Design review of the part built by this model. Coordinates are the model's own, in mm. A direction names the side the tool comes from. Give positions to 0.01 mm unless a question says otherwise; leave off trailing zeros. Loops run counter-clockwise (first coordinate to the right, second up) from the corner with the lowest first, then second, coordinate; pieces in that order, holes last. Notation, with made-up numbers: (12.5, 80) -> (47.5, 80) arc R14 cw to (47.5, 90) -> close; hole circle Ø5 at (45.5, 25.25). An arc over 180 degrees is marked (long way). Answer in a Markdown table with one row per item. Add a question column.
(1) Draft analysis for pull direction Y (two halves, no side actions). For faces 1 (the flat face through (3.763, 2.213, 2.442)), 2 (the cylindrical face through (-0.34, -1.55, 5.38)), 3 (the cylindrical face through (0.632, -1.525, 2.479)), 4 (the flat face through (0, -4.366, 2)), state which applies: +Y half, -Y half, draft (parallel to the pull), parting line (faces both ways), or undercut.
(2) For faces 5 (the flat face through (2, 0, 0)), 6 (the flat face through (0, -2, 5.715)), list the 3-axis set-ups (+Z, -Z, +X, -X, +Y, -Y) from which the entire face can be reached by the end or side of a thin tool; tool diameter is ignored.
(3) For line 1 (Y direction, x = 0, z = 2.1); line 2 (Y direction, x = 1.25, z = 5.45); line 3 (X direction, y = 1.5, z = 4.4), list the stretches that pass through material, from the lowest coordinate up.
(4) Consider section B-B on z = 0.55. Write out the cut boundary in (x, y), then the cut area to 3 significant figures.
(5) Consider section C-C on z = 5.55. Write out the cut boundary in (x, y) (1 decimal).
(6) For pin 1 (1.5 mm diameter, centred on x = 3.5, z = 2.5, fed in from +Y); pin 2 (1.7 mm diameter, centred on x = 0.5, y = 0, fed in from -Z); pin 3 (1 mm diameter, centred on y = -1.5, z = 1, fed in from -X); pin 4 (2.5 mm diameter, centred on x = 0, y = 0.5, fed in from +Z) (3 decimals), all flat-tipped, find the tip position at first contact; note any pin that passes through.
Autodesk Inventor part; units mm, degrees
ref_plane "YZ Plane" through (0, 0, 0) normal (1, 0, 0) x (0, 1, 0)
ref_plane "XZ Plane" through (0, 0, 0) normal (0, 1, 0) x (-1, 0, 0)
ref_plane "XY Plane" through (0, 0, 0) normal (0, 0, 1) x (1, 0, 0)
sketch "Sketch1" plane through (0, 0, 0) normal (0, 0, 1) x (1, 0, 0)
  line L0 (-2.5205, 4.3656) -> (2.5205, 4.3656)
  line L1 (2.5205, 4.3656) -> (5.041, 0)
  line L2 (5.041, 0) -> (2.5205, -4.3656)
  line L3 (2.5205, -4.3656) -> (-2.5205, -4.3656)
  line L4 (-2.5205, -4.3656) -> (-5.041, 0)
  line L5 (-5.041, 0) -> (-2.5205, 4.3656)
  point P0 (0, 0)
  point P1 (0, 0)
  dimension "d0" = 8.7312
extrude "Extrusion1" add sketch "Sketch1" along normal blind 4.953
sketch "Sketch2" plane through (0, 0, 0) normal (1, 0, 0) x (0, 1, 0)
  line L0 (4.3656, 4.953) -> (4.3656, 0) construction
  line L1 (4.3656, 0) -> (-4.3656, 0) construction
  line L2 (-4.3656, 0) -> (-4.3656, 4.953) construction
  line L3 (-4.3656, 4.953) -> (4.3656, 4.953) construction
  line L4 (0, 4.953) -> (0, 5.9436)
  line L5 (-4.3656, 4.953) -> (0, 4.953)
  arc A0 (-3.3782, 5.9436) -> (-4.3688, 4.953) centre (-3.3782, 4.953) ccw
  line L6 (-3.3782, 5.9436) -> (0, 5.9436)
  line L7 (0, 5.9436) -> (0, 4.953)
  line L8 (0, 4.953) -> (-4.3688, 4.953)
  point P0 (0, 0)
  dimension "d6" = 0.9906
  dimension "d7" = 3.3782
revolve "Revolution1" add sketch "Sketch2" angle 360 about axis through (0, 0, 4.953) along (0, 0, 1)
sketch "Sketch3" plane through (0, 0, 0) normal (0, 1, 0) x (-1, 0, 0)
  arc A0 (-3.3782, 5.9436) -> (-4.3688, 4.953) centre (-3.3782, 4.953) ccw construction
  line L0 (-3.3782, 5.9436) -> (3.3782, 5.9436) construction
  arc A1 (4.3688, 4.953) -> (3.3782, 5.9436) centre (3.3782, 4.953) ccw construction
  line L1 (4.3688, 4.953) -> (5.041, 4.953) construction
  line L2 (5.041, 4.953) -> (5.041, 0) construction
  line L3 (5.041, 0) -> (-5.041, 0) construction
  line L4 (-5.041, 0) -> (-5.041, 4.953) construction
  line L5 (-5.041, 4.953) -> (-4.3688, 4.953) construction
  line L6 (-4.3552, 4.953) -> (-5.041, 4.6482)
  line L7 (-5.041, 4.6482) -> (-5.041, 4.953)
  line L8 (-5.041, 4.953) -> (-4.3552, 4.953)
  line L9 (0, 0) -> (0, 7.4764) construction
  line L10 (-5.041, 0.3048) -> (-4.3552, 0)
  line L11 (-5.041, 0.3048) -> (-5.041, 0)
  line L12 (-5.041, 0) -> (-4.3552, 0)
  dimension "d9" = 0.6858
  dimension "d10" = 0.3048
  dimension "d11" = 0.3048
  dimension "d12" = 0.6858
revolve "Revolution2" cut sketch "Sketch3" angle 360 about axis through (0, 0, 0) along (0, 0, 1)
sketch "Sketch4" plane through (0, 0, 5.9436) normal (0, 0, 1) x (1, 0, 0)
  circle A0 centre (0, 0) radius 3.3782
hole "Hole1" at (0, 0, 5.9436) direction (0, 0, -1) diameter 3.302 end through all counterbore diameter 5.1054 counterbore depth 0.2286
sketch "Sketch5" plane through (0, 0, 5.715) normal (0, 0, 1) x (1, 0, 0)
  circle A0 centre (0, 0) radius 1.651
  circle A1 centre (0, 0) radius 1.5875
  dimension "d21" = 3.175
extrude "Extrusion2" add sketch "Sketch5" against normal blind 0.6858
equation "\"d6\" = d5"
properties part number "8-32 locknut" material "Aluminum 6061"
Values follow:
| question | item | result |
|---|---|---|
| 1 | face 1 | +Y half |
| 1 | face 2 | undercut |
| 1 | face 3 | undercut |
| 1 | face 4 | -Y half |
| 2 | face 5 | -Z, +X, -X, +Y, -Y |
| 2 | face 6 | +Z |
| 3 | line 1 | -4.37 to -1.65, 1.65 to 4.37 |
| 3 | line 2 | -4.05 to -0.98, 0.98 to 4.05 |
| 3 | line 3 | -4.17 to -0.69, 0.69 to 4.17 |
| 4 | outline | (-5.04, 0) -> (-2.52, -4.37) -> (2.52, -4.37) -> (5.04, 0) -> (2.52, 4.37) -> (-2.52, 4.37) -> close; hole circle Ø3.3 at (0, 0) |
| 4 | area | 57.5 mm2 |
| 5 | outline | circle Ø8.3 at (0, 0); hole circle Ø3.2 at (0, 0) |
| 6 | pin 1 | y = 3.97 |
| 6 | pin 2 | through |
| 6 | pin 3 | x = -4.46 |
| 6 | pin 4 | z = 5.715 |
